```python
from build123d import *

# Parameters (mm, degrees)
BOSS_EXTRUDE1_DEPTH = 10
SKETCH2_W           = 9.2
SKETCH2_H           = 9.2
CUT_EXTRUDE1_DEPTH  = 7
CUT_EXTRUDE2_DEPTH  = 11
BOSS_EXTRUDE2_DEPTH = 10
SKETCH5_R           = 1.9
CUT_EXTRUDE3_DEPTH  = 11


with BuildPart() as part:
    # Sketch1 → Boss-Extrude1 (new body)
    with BuildSketch(Plane(origin=(0, 0, 0), x_dir=(1, 0, 0), z_dir=(0, 1, 0))):
        Polygon((0, 0), (75, 0), (37.5, 64.951905284), align=None)
    extrude(amount=BOSS_EXTRUDE1_DEPTH)

    # Sketch2 → Cut-Extrude1 (cut)
    with BuildSketch(Plane(origin=(0, 10, 0), x_dir=(1, 0, 0), z_dir=(0, 1, 0))):
        with Locations((55, 12.6)):
            Rectangle(SKETCH2_W, SKETCH2_H)
        with Locations((20, 12.6)):
            Rectangle(SKETCH2_W, SKETCH2_H)
    extrude(amount=-CUT_EXTRUDE1_DEPTH, mode=Mode.SUBTRACT)

    # Sketch3 → Cut-Extrude2 (cut, through all)
    with BuildSketch(Plane(origin=(0, 10, 0), x_dir=(1, 0, 0), z_dir=(0, 1, 0))):
        Polygon((18.75, 32.475952642), (26.3, 45.552936239), (31.063139721, 42.802936239), (18.463139721, 20.979096064), (13.7, 23.729096064), align=None)
    extrude(amount=-CUT_EXTRUDE2_DEPTH, mode=Mode.SUBTRACT)

    # Sketch4 → Boss-Extrude2 (add)
    with BuildSketch(Plane(origin=(0, 10, 0), x_dir=(1, 0, 0), z_dir=(0, 1, 0))):
        Polygon((56.25, 32.475952642), (48.75, 45.466333699), (53.080127019, 47.966333699), (65.580127019, 26.315698604), (61.25, 23.815698604), align=None)
    extrude(amount=-BOSS_EXTRUDE2_DEPTH)

    # Sketch5 → Cut-Extrude3 (cut, through all)
    with BuildSketch(Plane(origin=(0, 10, 0), x_dir=(1, 0, 0), z_dir=(0, 1, 0))):
        with Locations((37.5, 39.951905284)):
            Circle(SKETCH5_R)
        with BuildLine():
            Line((30, 51.961524227), (37.5, 64.951905284))
            Line((37.5, 64.951905284), (45, 51.961524227))
            ThreePointArc((45, 51.961524227), (37.5, 49.951905284), (30, 51.961524227))
        make_face()
    extrude(amount=-CUT_EXTRUDE3_DEPTH, mode=Mode.SUBTRACT)


solid = part.part
```
The listing builds one solid part. Answer for the finished solid, in the listing's coordinates (mm). A direction names the side the tool comes from. Round coordinates to 2 decimals unless told otherwise and drop trailing zeros. Loops run counter-clockwise (first coordinate to the right, second up) from the corner with the lowest first, then second, coordinate; pieces in that order, holes last.
Q1. Section C-C, the plane x = 19.5 is taken. Determine the outline of the cut face in (y, z) (3 decimals), then the cut area to 3 significant figures.
Q2. Section A-A, the plane x = 37.5 is taken. Determine the outline of the cut face in (y, z), then the cut area to 3 significant figures.
Q3. For a pull along X with two mould halves and no side action, classify faces 1 (the face through (28.648, 5.07, -44.197)), 2 (the face through (37.61, 5.07, -49.952)), 3 (the face through (15.4, 7, -13)), 4 (the face through (37, 0, -21)) as released by +X, released by -X, zero draft, split by the parting line, or undercut.
Q4. Which of the six approach directions +Z, -Z, +X, -X, +Y, -Y give full straight-line access (tool end or side, diameter ignored) to faces 5 (the face through (39.312, 5.07, -40.523)), 6 (the face through (16.115, 5.07, -22.335)), 7 (the face through (63.445, 5.07, -25.083)), 8 (the face through (55, 7, -17.2))?
Q5. Section D-D, the plane z = -13 is taken. Determine the outline of the cut face in (x, y), then the cut area to 3 significant figures.
Q6. Find the intervals of material crossed by line 1 (Z direction, x = 37.5, y = 5.5); line 2 (X direction, y = 8.25, z = -16); line 3 (X direction, y = 4.25, z = -14.5), in increasing order.
Q7. Section B-B, the plane y = 6 is taken. Determine the outline of the cut face in (x, z), then the cut area to 3 significant figures.
Q8. Given pin 1 Ø5.5 at (y, z) = (7, -14) entering from -X; pin 2 Ø10 at (x, z) = (38.5, -10) entering from -Y; pin 3 Ø2 at (y, z) = (7, -13.5) entering from +X; pin 4 Ø3.5 at (x, y) = (55.5, 6.5) entering from -Z, each flat-ended and moving along its own axis, determine where each tip first touches the part or whether it passes through.
Completed:
1. outline: (0, -22.775) - (10, -22.775) - (10, -17.2) - (3, -17.2) - (3, -8) - (10, -8) - (10, 0) - (0, 0) - close
1. area: 163 mm2
2. outline: (0, -49.95) - (10, -49.95) - (10, -41.85) - (0, -41.85) - close; (0, -38.05) - (10, -38.05) - (10, 0) - (0, 0) - close
2. area: 462 mm2
3. face 1: released by -X
3. face 2: undercut
3. face 3: undercut
3. face 4: zero draft
4. face 5: +Y, -Y
4. face 6: -Z, +Y, -Y
4. face 7: +X, +Y, -Y
4. face 8: +Y
5. outline: (7.51, 0) - (67.49, 0) - (67.49, 10) - (59.6, 10) - (59.6, 3) - (50.4, 3) - (50.4, 10) - (24.6, 10) - (24.6, 3) - (15.4, 3) - (15.4, 10) - (7.51, 10) - close
5. area: 471 mm2
6. line 1: z = -49.95 to -41.85, -38.05 to 0
6. line 2: x = 9.24 to 15.4, 24.6 to 50.4, 59.6 to 65.76
6. line 3: x = 8.37 to 15.4, 24.6 to 50.4, 59.6 to 66.63
7. outline: (0, 0) - (13.7, -23.73) - (18.46, -20.98) - (31.06, -42.8) - (26.3, -45.55) - (30, -51.96) arc R15 cw to (45, -51.96) - (48.75, -45.47) - (53.08, -47.97) - (65.58, -26.32) - (61.25, -23.82) - (75, 0) - close; hole (15.4, -17.2) - (24.6, -17.2) - (24.6, -8) - (15.4, -8) - close; hole circle Ø3.8 at (37.5, -39.95); hole (50.4, -17.2) - (59.6, -17.2) - (59.6, -8) - (50.4, -8) - close
7. area: 2,120 mm2
8. pin 1: stops at x = 6.5
8. pin 2: stops at y = 0
8. pin 3: stops at x = 67.78
8. pin 4: stops at z = -46.81
